Part print with two shaded views. Sizes in mm from the minimum x, y, z corner. A direction names the side the tool comes from. Round coordinates to 2 decimals unless told otherwise and drop trailing zeros. Write each loop counter-clockwise with the first axis right and the second up, starting at its lowest first coordinate (ties: lowest second). Pieces come first, ordered by that corner, then holes. Notation, with made-up numbers: (6.25, 84.25) -> (53.25, 84.25) arc R14 ccw to (53.25, 106.25) -> close; hole circle Ø9 at (64.5, -11.75). An arc over 180 degrees is marked (long way). Return JSON: item names as keys, results as strings. Group by question number.
(1) Drill centre lines: L1, parallel to X at y = 9.5, z = 43.5; L2, parallel to Z at x = 40.5, y = 38; L3, parallel to X at y = 39, z = 46.5. Where is each one in solid material? Low to high. Write a range as from..to.
(2) Saw through at D-D (y = 33.5). List the corners of the cut face in (x, z) (1 decimal), plus the area to 3 significant figures.
(3) Saw through at B-B (x = 39). List the corners of the cut face in (y, z).
(4) Tool access for the marked faces 1 and 2: list every direction of +Z, -Z, +X, -X, +Y, -Y with a clear straight run to the whole face (end or side of a thin tool).
(5) Saw through at A-A (y = 23). List the corners of the cut face in (x, z), plus the area to 3 significant figures.
(6) Drop flat-ended pins along their axis: pin 1 Ø5.5 at (y, z) = (67, 5) entering from -X; pin 2 Ø6.5 at (x, y) = (5.5, 55) entering from -Z; pin 3 Ø6.5 at (x, z) = (15, 64.5) entering from +Y. Give the stop position or say it passes through.
(7) Saw through at C-C (z = 56). List the corners of the cut face in (x, y), plus the area to 3 significant figures.
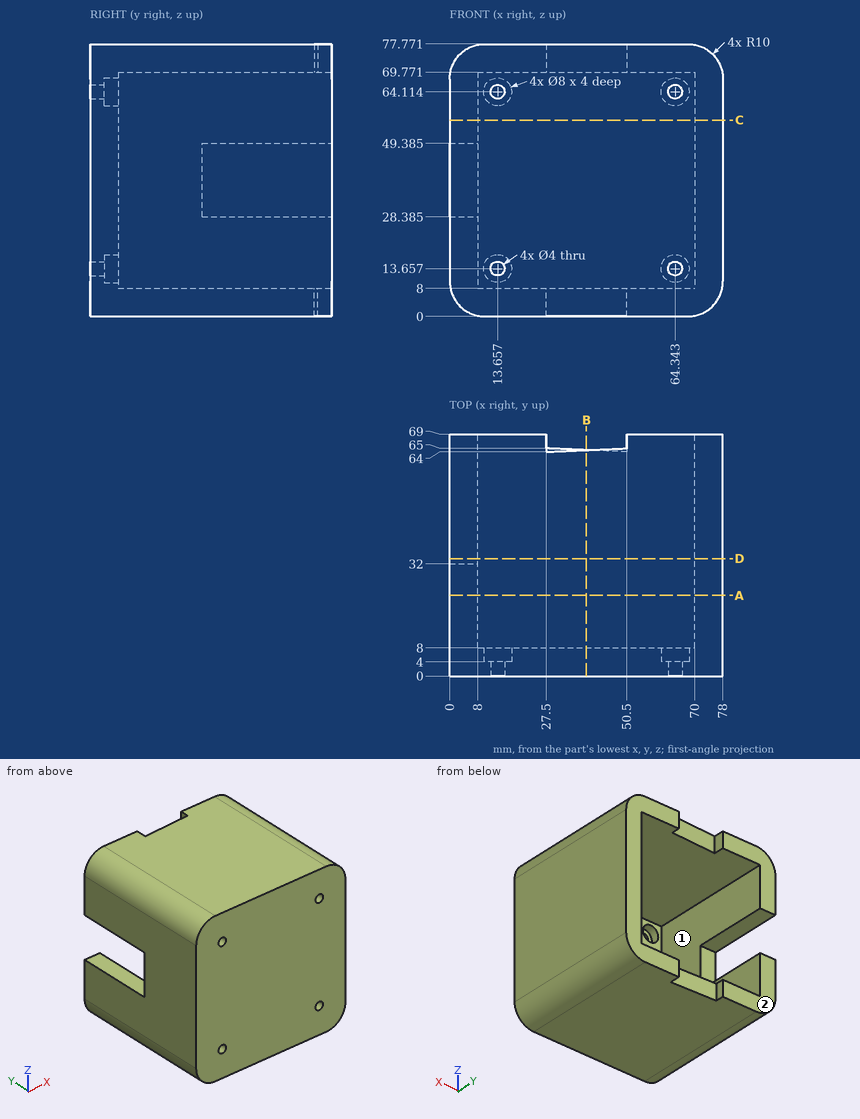
Computed values:
{
 "1": {"L1": "0..8, 70..78", "L2": "0..8, 69.77..77.77", "L3": "70..78"},
 "2": {"outline": "(0, 10) arc R10 ccw to (10, 0) -> (68, 0) arc R10 ccw to (78, 10) -> (78, 67.8) arc R10 ccw to (68, 77.8) -> (10, 77.8) arc R10 ccw to (0, 67.8) -> (0, 49.4) -> (8, 49.4) -> (8, 69.8) -> (70, 69.8) -> (70, 8) -> (8, 8) -> (8, 28.4) -> (0, 28.4) -> close", "area": "1,980 mm2"},
 "3": {"outline": "(0, 0) -> (64.5, 0) -> (64.5, 8) -> (8, 8) -> (8, 69.77) -> (64.5, 69.77) -> (64.5, 77.77) -> (0, 77.77) -> close"},
 "4": {"face 1": "+Y", "face 2": "+Z, -Z, +X, -X, +Y"},
 "5": {"outline": "(0, 10) arc R10 ccw to (10, 0) -> (68, 0) arc R10 ccw to (78, 10) -> (78, 67.77) arc R10 ccw to (68, 77.77) -> (10, 77.77) arc R10 ccw to (0, 67.77) -> close; hole (8, 8) -> (70, 8) -> (70, 69.77) -> (8, 69.77) -> close", "area": "2,150 mm2"},
 "6": {"pin 1": "x = 0.26", "pin 2": "z = 0.08", "pin 3": "y = 8"},
 "7": {"outline": "(0, 0) -> (78, 0) -> (78, 69) -> (70, 69) -> (70, 8) -> (8, 8) -> (8, 69) -> (0, 69) -> close", "area": "1,600 mm2"}
}
